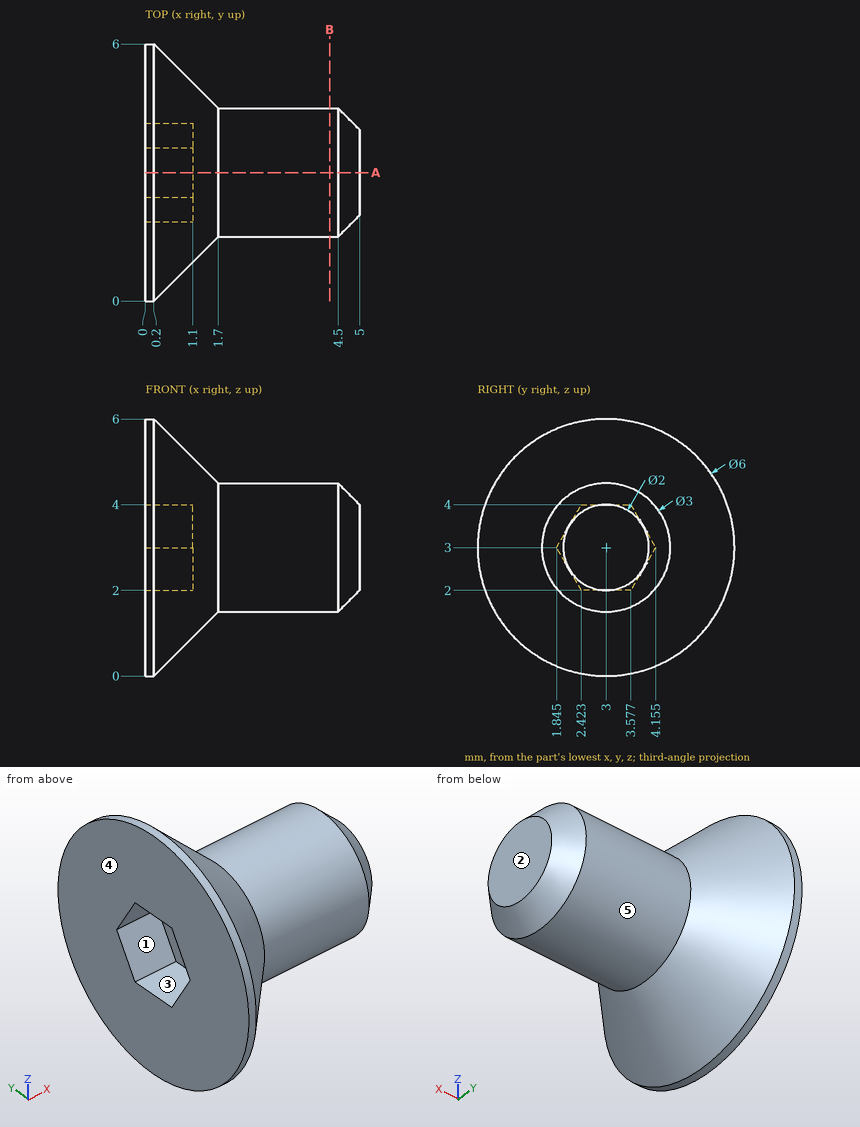
For this review, use the dimensioned drawing (mm, ordinates from the lowest corner) and the shaded views. A direction names the side the tool comes from. Give positions to 0.01 mm unless a question says otherwise; leave off trailing zeros. Order: outer loops, then holes, each group sorted by start corner. A loop starts at its lowest first (then second) coordinate and runs counter-clockwise, first axis right, second up. Notation, with made-up numbers: M 31.25,-13 L 82.25,-13 A20 ccw 82.25,17 Z; hole C 52.25,58.5 d11. An arc over 180 degrees is marked long. Use one line per item in the form item = value. Start each with the question number.
Item 1: We need section A-A on y = 3. Give the boundary of the cut face in (x, z), plus the area to 3 significant figures.
Item 2: To check wall thickness, follow line 1 along X through (y, z) = (3.5, 3.05); line 2 along Z through (x, y) = (0.75, 2.2) (1 decimal); line 3 along Z through (x, y) = (0.75, 3.25). State the ranges of each line that lie inside material, in increasing order. Write a range as from..to.
Item 3: For the marked faces 1 and 2, list the 3-axis set-ups (+Z, -Z, +X, -X, +Y, -Y) from which the entire face can be reached by the end or side of a thin tool; tool diameter is ignored.
Item 4: Insertion check: pin 1 Ø1.5 at (x, z) = (0.5, 5) entering from -Y; pin 2 Ø3 at (x, y) = (2.5, 5) entering from -Z; pin 3 Ø0.6 at (y, z) = (3, 3) entering from -X; pin 4 Ø0.9 at (x, y) = (0.5, 3) entering from +Z. Each pin has a flat end and moves straight along its axis. Give the tip position at first contact, or say it passes through.
Item 5: We need section B-B on x = 4.3. Give the boundary of the cut face in (y, z).
Item 6: The part is to be moulded in two halves that separate along Y. For the marked faces 3, 4 and 5, say which applies: pulls with the +Y half, pulls with the -Y half, needs draft (parallel to the pull), parting line crosses it, or undercut.
Completed:
q1.outline = M 0,0 L 0.2,0 L 1.7,1.5 L 4.5,1.5 L 5,2 L 5,4 L 4.5,4.5 L 1.7,4.5 L 0.2,6 L 0,6 L 0,4 L 1.1,4 L 1.1,2 L 0,2 Z
q1.area = 15.4 mm²
q2.line_1 = 1.1..5
q2.line_2 = 0.7..2.4, 3.6..5.3
q2.line_3 = 0.56..2, 4..5.44
q3.face_1 = -X
q3.face_2 = +Z, -Z, +X, +Y, -Y
q4.pin_1 = 0.3
q4.pin_2 = 1.44
q4.pin_3 = 1.1
q4.pin_4 = 6
q5.outline = C 3,3 d3
q6.face_3 = undercut
q6.face_4 = needs draft
q6.face_5 = parting line crosses it
